from build123d import *

# Parameters (mm, degrees)
SKETCH1_W                      = 110
SKETCH1_H                      = 90
BOSS_EXTRUDE1_DEPTH            = 2.5
M3_CLEARANCE_HOLE1_D           = 3.4
M3_CLEARANCE_HOLE1_DEPTH       = 5
SKETCH5_W                      = 110
SKETCH5_H                      = 6.35
BOSS_EXTRUDE2_DEPTH            = 25
BOSS_EXTRUDE2_DEPTH_BACK       = 2.5
CBORE_FOR_M3_SHCS1_D           = 3.4
CBORE_FOR_M3_SHCS1_DEPTH       = 6.35
CBORE_FOR_M3_SHCS1_CBORE_D     = 6.5
CBORE_FOR_M3_SHCS1_CBORE_DEPTH = 3
CUT_EXTRUDE1_DEPTH             = 6
BOSS_EXTRUDE4_DEPTH            = 5
FILLET1_R                      = 5
FILLET2_R                      = 5


with BuildPart() as part:
    # Sketch1 → Boss-Extrude1 (new body, symmetric)
    with BuildSketch(Plane(origin=(0, 0, 0), x_dir=(1, 0, 0), z_dir=(0, 1, 0))):
        with Locations((55, -45)):
            Rectangle(SKETCH1_W, SKETCH1_H)
    extrude(amount=BOSS_EXTRUDE1_DEPTH, both=True)

    # M3 Clearance Hole1
    with Locations(Plane(origin=(0, 2.5, 0), x_dir=(1, 0, 0), z_dir=(0, 1, 0))):
        with Locations((13.4, -77.55755), (96.6, -12.44245), (96.6, -77.55755), (13.4, -12.44245)):
            Hole(M3_CLEARANCE_HOLE1_D / 2, depth=M3_CLEARANCE_HOLE1_DEPTH)

    # Sketch5 → Boss-Extrude2 (add, two sides)
    with BuildSketch(Plane(origin=(0, 0, 0), x_dir=(1, 0, 0), z_dir=(0, 1, 0))) as boss_extrude2_sk:
        with Locations((55, -93.175)):
            Rectangle(SKETCH5_W, SKETCH5_H)
    extrude(amount=BOSS_EXTRUDE2_DEPTH)
    extrude(boss_extrude2_sk.sketch, amount=-BOSS_EXTRUDE2_DEPTH_BACK)

    # CBORE for M3 SHCS1
    with Locations(Plane(origin=(0, 0, 90), x_dir=(-1, 0, 0), z_dir=(0, 0, -1))):
        with Locations((-80, 13.75), (-30, 13.75)):
            CounterBoreHole(CBORE_FOR_M3_SHCS1_D / 2, CBORE_FOR_M3_SHCS1_CBORE_D / 2, CBORE_FOR_M3_SHCS1_CBORE_DEPTH, depth=CBORE_FOR_M3_SHCS1_DEPTH)

    # Sketch8 → Cut-Extrude1 (cut, through all)
    with BuildSketch(Plane(origin=(0, 2.5, 0), x_dir=(1, 0, 0), z_dir=(0, 1, 0))):
        Polygon((17.9, -9.9), (92.1, -9.9), (92.1, -16.12616408), (100.1, -16.12616408), (100.1, -73.87383592), (92.1, -73.87383592), (92.1, -80.1), (17.9, -80.1), (17.9, -73.87383592), (9.9, -73.87383592), (9.9, -16.12616408), (17.9, -16.12616408), align=None)
    extrude(amount=-CUT_EXTRUDE1_DEPTH, mode=Mode.SUBTRACT)

    # Sketch10 → Boss-Extrude4 (add, through all)
    with BuildSketch(Plane(origin=(0, 2.5, 0), x_dir=(1, 0, 0), z_dir=(0, 1, 0))):
        Polygon((40.1, -9.9), (92.1, -9.9), (92.1, -16.12616408), (100.1, -16.12616408), (100.1, -73.87383592), (92.1, -73.87383592), (92.1, -80.1), (40.1, -80.1), align=None)
    extrude(amount=-BOSS_EXTRUDE4_DEPTH)

    # Fillet1
    fillet1_edges = [part.edges().sort_by_distance(p)[0] for p in [
        (0, 0, 0),
        (110, 0, 0),
    ]]
    fillet(fillet1_edges, radius=FILLET1_R)

    # Fillet2
    fillet2_edges = [part.edges().sort_by_distance(p)[0] for p in [
        (55, 2.5, 90),
    ]]
    fillet(fillet2_edges, radius=FILLET2_R)


solid = part.part
Geometry check sheet. Reference: the model listing, model coordinates, mm. A direction names the side the tool comes from. Give positions to 0.01 mm unless a question says otherwise; leave off trailing zeros. Loops run counter-clockwise (first coordinate to the right, second up) from the corner with the lowest first, then second, coordinate; pieces in that order, holes last. Notation, with made-up numbers: M -2,-30 L 32,-30 A14 cw 32,-10 Z; hole C 66,29.25 d3. An arc over 180 degrees is marked long. Answer as a JSON object with one key per item and string values. Group by question number.
Item 1: Sectioned sample at D-D on y = 13.75. Record the boundary of the cut face in (x, z), plus the area to 3 significant figures.
Item 2: Sectioned sample at B-B on z = 72. Record the boundary of the cut face in (x, y).
Item 3: Access from +Z, -Z, +X, -X, +Y, -Y to the whole of each face (thin tool, end or side, straight path). Record for faces 1 (the cylindrical face through (31.57, 13.1, 94.7)), 2 (the flat face through (14, 0, 16.126)), 3 (the cylindrical face through (83.247, 13.893, 91.479)).
Item 4: Sectioned sample at A-A on x = 80. Record the boundary of the cut face in (y, z).
Item 5: Material ranges on L1, parallel to Z at x = 96.6, y = -0.7; L2, parallel to Z at x = 13.4, y = -0.6; L3, parallel to Z at x = 20, y = -1, recorded low to high.
Item 6: Gauge pin test, flat ends, axial feed: pin 1 (6 mm diameter, centred on y = 7, z = 80, fed in from -X); pin 2 (5.5 mm diameter, centred on x = 80, y = 13.75, fed in from -Z); pin 3 (1.5 mm diameter, centred on x = 56.5, y = 21, fed in from -Z). Record the tip position at first contact, or that the pin passes through.
Item 7: Mould release check, pull along X, two halves, no side actions. Record for faces 4 (the flat face through (29, 12, 93)), 5 (the flat face through (29, 0, 80.1)), 6 (the flat face through (110, 1, 61)), 7 (the flat face through (54, 25, 93)): pulls with the +X half, pulls with the -X half, needs draft (parallel to the pull), parting line crosses it, or undercut.
Item 8: Sectioned sample at C-C on x = 30. Record the boundary of the cut face in (y, z), plus the area to 3 significant figures.
Findings below:
{
 "1": {"outline": "M 0,90 L 26.75,90 L 26.75,93 L 28.3,93 L 28.3,96.35 L 0,96.35 Z; M 31.7,93 L 33.25,93 L 33.25,90 L 76.75,90 L 76.75,93 L 78.3,93 L 78.3,96.35 L 31.7,96.35 Z; M 81.7,93 L 83.25,93 L 83.25,90 L 110,90 L 110,96.35 L 81.7,96.35 Z", "area": "637 mm2"},
 "2": {"outline": "M 0,-2.5 L 9.9,-2.5 L 9.9,2.5 L 0,2.5 Z; M 40.1,-2.5 L 110,-2.5 L 110,2.5 L 40.1,2.5 Z"},
 "3": {"face 1": "+Z, -Z", "face 2": "+Y, -Y", "face 3": "-Z"},
 "4": {"outline": "M -2.5,0 L 2.5,0 L 2.5,85 A5 cw 7.5,90 L 10.5,90 L 10.5,93 L 12.05,93 L 12.05,96.35 L -2.5,96.35 Z; M 15.45,93 L 17,93 L 17,90 L 25,90 L 25,96.35 L 15.45,96.35 Z"},
 "5": {"L1": "0 to 10.74, 14.14 to 75.86, 79.26 to 96.35", "L2": "0 to 10.74, 14.14 to 16.13, 73.87 to 75.86, 79.26 to 96.35", "L3": "0 to 9.9, 80.1 to 96.35"},
 "6": {"pin 1": "through", "pin 2": "z = 93", "pin 3": "z = 90"},
 "7": {"face 4": "undercut", "face 5": "undercut", "face 6": "pulls with the +X half", "face 7": "needs draft"},
 "8": {"outline": "M -2.5,0 L 2.5,0 L 2.5,9.9 L -2.5,9.9 Z; M -2.5,80.1 L 2.5,80.1 L 2.5,85 A5 cw 7.5,90 L 10.5,90 L 10.5,93 L 12.05,93 L 12.05,96.35 L -2.5,96.35 Z; M 15.45,93 L 17,93 L 17,90 L 25,90 L 25,96.35 L 15.45,96.35 Z", "area": "248 mm2"}
}
